Read the model definition and answer for the solid it produces. Units are mm, in the model's axes. Give positions to 0.01 mm unless a question says otherwise; leave off trailing zeros. Write each loop counter-clockwise with the first axis right and the second up, starting at its lowest first coordinate (ties: lowest second). Pieces come first, ordered by that corner, then holes.
Autodesk Inventor part; units mm, degrees
ref_plane "YZ Plane" through (0, 0, 0) normal (1, 0, 0) x (0, 1, 0)
ref_plane "XZ Plane" through (0, 0, 0) normal (0, 1, 0) x (-1, 0, 0)
ref_plane "XY Plane" through (0, 0, 0) normal (0, 0, 1) x (1, 0, 0)
sketch "Sketch1" plane through (0, 0, 0) normal (0, 0, 1) x (1, 0, 0)
  line L0 (0, 0) -> (184.15, 0)
  line L1 (184.15, 94.488) -> (0, 94.488)
  line L2 (190.5, 47.244) -> (190.5, 66.294)
  line L3 (190.5, 66.294) -> (184.15, 66.294)
  line L4 (190.5, 47.244) -> (190.5, 28.194)
  line L5 (190.5, 28.194) -> (184.15, 28.194)
  line L6 (-6.35, 47.244) -> (-6.35, 66.294)
  line L7 (-6.35, 66.294) -> (0, 66.294)
  line L8 (-6.35, 47.244) -> (-6.35, 28.194)
  line L9 (-6.35, 28.194) -> (0, 28.194)
  line L10 (0, 94.488) -> (0, 66.294)
  line L11 (0, 28.194) -> (0, 0)
  line L12 (184.15, 0) -> (184.15, 28.194)
  line L13 (184.15, 66.294) -> (184.15, 94.488)
  dimension "d0" = 184.15
extrude "Extrusion1" add sketch "Sketch1" along normal blind 5.5563
sketch "Sketch2" plane through (0, 0, 0) normal (0, 0, -1) x (-1, 0, 0)
  line L0 (0, 0) -> (0, 6.35)
  line L1 (0, 28.194) -> (0, 0)
  line L2 (0, 6.35) -> (-6.35, 6.35)
  line L3 (-6.35, 6.35) -> (-6.35, 0)
  line L4 (0, 6.35) -> (0, 0)
  line L5 (0, 0) -> (-184.15, 0)
  line L6 (-6.35, 0) -> (0, 0)
extrude "Extrusion2" cut sketch "Sketch2" against normal blind 6.35
properties part number "lower_front_wall"
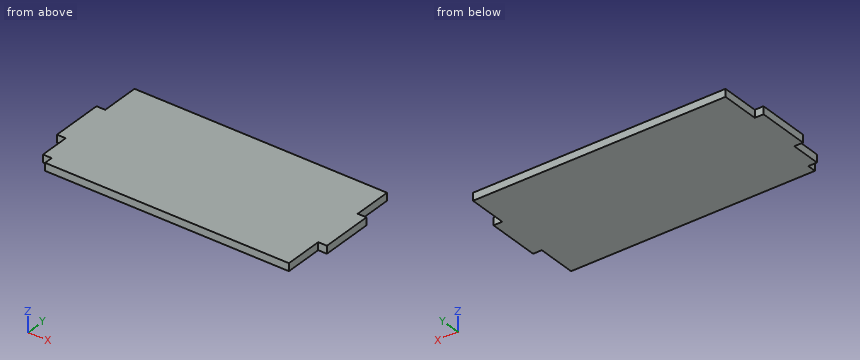
Item 1: Section A-A (z = 2.7) is taken. Write down the section's boundary in (x, y).
Result set:
outline: (-6.35, 28.19) - (0, 28.19) - (0, 6.35) - (6.35, 6.35) - (6.35, 0) - (184.15, 0) - (184.15, 28.19) - (190.5, 28.19) - (190.5, 66.29) - (184.15, 66.29) - (184.15, 94.49) - (0, 94.49) - (0, 66.29) - (-6.35, 66.29) - close
Item 2: Section B-B (y = 19) is taken. Write down the section's boundary in (x, z), and give its area (3 significant figures).
Result set:
outline: (0, 0) - (184.15, 0) - (184.15, 5.56) - (0, 5.56) - close
area: 1,020 mm2
Item 3: Find the intervals of material crossed by line 1 along X through (y, z) = (17.5, 2.45), in increasing order.
Result set:
line 1: x = 0 to 184.15
Item 4: Each of these flat-tipped pins is pushed along its axis until it touches: pin 1 Ø1.7 at (x, z) = (4, 1.5) entering from -Y; pin 2 Ø3 at (y, z) = (85, 2.5) entering from +X; pin 3 Ø1.7 at (x, z) = (188, 2) entering from +Y. Where does it stop, or does it pass through?
Result set:
pin 1: stops at y = 6.35
pin 2: stops at x = 184.15
pin 3: stops at y = 66.29
